Autodesk Inventor part; units mm, degrees
ref_plane "bnt_nut_1_XY" through (0, 0, 0) normal (1, 0, 0) x (0, 0, -1)
ref_plane "bnt_nut_1_YZ" through (0, 0, 0) normal (0, 0, -1) x (0, 1, 0)
ref_plane "bnt_nut_1_ZX" through (0, 0, 0) normal (0, 1, 0) x (1, 0, 0)
sketch "Sketch_1" plane through (0, 0, 0) normal (1, 0, 0) x (0, 1, 0)
  line L0 (17, 24) -> (7, 24)
  line L1 (7, 24) -> (6, 23)
  line L2 (6, 23) -> (-12, 23)
  line L3 (-19, 16) -> (-19, -16)
  line L4 (-12, -23) -> (6, -23)
  line L5 (6, -23) -> (7, -24)
  line L6 (7, -24) -> (17, -24)
  line L7 (17, -24) -> (17, -11)
  line L8 (17, -11) -> (16, -10)
  line L9 (16, -10) -> (16, 10)
  line L10 (16, 10) -> (17, 11)
  line L11 (17, 11) -> (17, 24)
  circle A0 centre (0, 0) radius 10
  line L12 (16, 0) -> (0, 0) construction
  line L13 (-12, -23) -> (-19, -16)
  line L14 (-12, 23) -> (-19, 16)
  line L15 (0, 0) -> (-19, 0) construction
  line L16 (6, 23) -> (6, -23) construction
  dimension "d39" = 20
  dimension "d41" = 46
  dimension "d43" = 23
  dimension "d45" = 1
  dimension "d46" = 48
  dimension "d47" = 1
  dimension "d48" = 36
  dimension "d49" = 10
  dimension "d50" = 10
  dimension "d51" = 20
  dimension "d52" = 13
  dimension "d53" = 13
  dimension "d54" = 32
  dimension "d55" = 16
  dimension "d56" = 135
  dimension "d57" = 18
  dimension "d58" = 18
extrude "Extrusion1" add sketch "Sketch_1" along normal blind 38
sketch "Sketch_2" plane through (29, 0, 0) normal (0.682, 0, 0.7314) x (0.7314, 0, -0.682)
  line L0 (-29, -24.55) -> (-4.4539, -24.55)
  arc A0 (-4.4539, -24.55) -> (4.4539, -24.55) centre (0, -23.4) ccw
  line L1 (4.4539, -24.55) -> (29, -24.55)
  line L2 (29, -24.55) -> (29, -23.4)
  line L3 (29, -23.4) -> (-29, -23.4)
  line L4 (-29, -23.4) -> (-29, -24.55)
  dimension "d33" = 58
  dimension "d34" = 1.15
  dimension "d35" = 24.5461
  dimension "d36" = 4.6
  dimension "d37" = 24.5461
  dimension "d38" = 1.15
extrude "Extrusion2" [suppressed]
sketch "Sketch_3" plane through (0, -23.4, 0) normal (0, 1, 0) x (1, 0, 0)
  line L0 (-29, -58) -> (87, -58)
  line L1 (87, -58) -> (87, 58)
  line L2 (87, 58) -> (-29, 58)
  line L3 (-29, 58) -> (-29, -58)
  line L4 (9.6667, -9.44) -> (48.3333, -9.44)
  line L5 (48.3333, -9.44) -> (48.3333, 9.44)
  line L6 (48.3333, 9.44) -> (9.6667, 9.44)
  line L7 (9.6667, 9.44) -> (9.6667, -9.44)
extrude "Extrusion3" [suppressed]
sketch "Sketch_4" plane through (0, 0, 0) normal (0, 0, 1) x (1, 0, 0)
  line L0 (13.4367, -26.15) -> (13.4367, -24.55)
  line L1 (13.4367, -24.55) -> (15.4367, -24.55)
  line L2 (15.4367, -24.55) -> (15.4367, -25.75)
  arc A0 (15.0367, -26.15) -> (15.4367, -25.75) centre (15.0367, -25.75) ccw
  line L3 (15.0367, -26.15) -> (13.4367, -26.15)
  line L4 (13.4367, -26.15) -> (13.4367, -24.55)
revolve "Revolution1" [suppressed]
sketch "Sketch_5" plane through (0, 0, 0) normal (0, 0, 1) x (1, 0, 0)
  line L0 (44.5633, -26.15) -> (44.5633, -24.55)
  line L1 (44.5633, -24.55) -> (46.5633, -24.55)
  line L2 (46.5633, -24.55) -> (46.5633, -25.75)
  arc A0 (46.1633, -26.15) -> (46.5633, -25.75) centre (46.1633, -25.75) ccw
  line L3 (46.1633, -26.15) -> (44.5633, -26.15)
  line L4 (44.5633, -26.15) -> (44.5633, -24.55)
revolve "Revolution2" [suppressed]
sketch "Sketch_6" plane through (0, -26.15, 0) normal (0, 1, 0) x (1, 0, 0)
  line L0 (43.5633, 0.15) -> (43.5633, -0.15)
  line L1 (43.5633, -0.15) -> (44.4133, -0.15)
  line L2 (44.4133, -0.15) -> (44.4133, -1)
  line L3 (44.4133, -1) -> (44.7133, -1)
  line L4 (44.7133, -1) -> (44.7133, -0.15)
  line L5 (44.7133, -0.15) -> (45.5633, -0.15)
  line L6 (45.5633, -0.15) -> (45.5633, 0.15)
  line L7 (45.5633, 0.15) -> (44.7133, 0.15)
  line L8 (44.7133, 0.15) -> (44.7133, 1)
  line L9 (44.7133, 1) -> (44.4133, 1)
  line L10 (44.4133, 1) -> (44.4133, 0.15)
  line L11 (44.4133, 0.15) -> (43.5633, 0.15)
extrude "Extrusion4" [suppressed]
sketch "Sketch_7" plane through (0, -26.15, 0) normal (0, 1, 0) x (1, 0, 0)
  line L0 (12.4367, 0.15) -> (12.4367, -0.15)
  line L1 (12.4367, -0.15) -> (13.2867, -0.15)
  line L2 (13.2867, -0.15) -> (13.2867, -1)
  line L3 (13.2867, -1) -> (13.5867, -1)
  line L4 (13.5867, -1) -> (13.5867, -0.15)
  line L5 (13.5867, -0.15) -> (14.4367, -0.15)
  line L6 (14.4367, -0.15) -> (14.4367, 0.15)
  line L7 (14.4367, 0.15) -> (13.5867, 0.15)
  line L8 (13.5867, 0.15) -> (13.5867, 1)
  line L9 (13.5867, 1) -> (13.2867, 1)
  line L10 (13.2867, 1) -> (13.2867, 0.15)
  line L11 (13.2867, 0.15) -> (12.4367, 0.15)
extrude "Extrusion5" [suppressed]
sketch "Sketch8" plane through (0, -12, 23) normal (0, 0, 1) x (1, 0, 0)
  line L0 (0, 18) -> (0, 0)
  point P0 (7, 11.14)
  dimension "d61" = 7
hole "Hole1" at (7, -0.86, 23) direction (0, 0, -1) diameter 4.917 depth 14.1406 tip angle 120 countersink diameter 6 countersink angle 90
sketch "Sketch9" plane through (0, 17, -11) normal (0, 1, 0) x (1, 0, 0)
  line L0 (0, 13) -> (0, 0)
  line L1 (0, 13) -> (38, 13)
  point P0 (8, 7)
  dimension "d59" = 8
  dimension "d60" = 6
hole "Hole2" at (8, 17, -18) direction (0, -1, 0) diameter 4.134 depth 13 tip angle 120 countersink diameter 6 countersink angle 90
pattern_linear "Rectangular Pattern1" count 2 spacing 22 along (1, 0, 0) count 2 spacing 35 along (0, 0, 1) of "Hole2"
ref_plane "bnt_nut_1_XY" through (0, 0, 0) normal (1, 0, 0) x (0, 0, -1)
ref_plane "bnt_nut_1_YZ" through (0, 0, 0) normal (0, 0, -1) x (0, 1, 0)
ref_plane "bnt_nut_1_ZX" through (0, 0, 0) normal (0, 1, 0) x (1, 0, 0)
sketch "Sketch10" plane through (38, -23.4, -9.44) normal (0, 0, -1) x (-1, 0, 0)
  point P0 (38, 23.4)
sketch "Sketch11" plane through (38, 0, 0) normal (1, 0, 0) x (0, 0, -1)
  circle A0 centre (0, 0) radius 15.5
  dimension "d62" = 31
properties part number "BNT 2010-2.6 Nut"
CAD build for the part. Positions are in the model's coordinates, mm. A direction names the side the tool comes from. Round coordinates to 2 decimals unless told otherwise and drop trailing zeros. Write each loop counter-clockwise with the first axis right and the second up, starting at its lowest first coordinate (ties: lowest second). Pieces come first, ordered by that corner, then holes. Notation, with made-up numbers: (28.5, 65) -> (37.5, 65) arc R28 ccw to (37.5, 98) -> close; hole circle Ø5 at (5.5, 39.5). An arc over 180 degrees is marked (long way). Answer in a Markdown table with one row per item. Add a question column.
Item 1: Saw through at B-B, the plane x = 25. Write the cut outline in (y, z).
Item 2: Saw through at A-A, the plane z = 0. Write the cut outline in (x, y).
Item 3: Which spindle directions (+Z, -Z, +X, -X, +Y, -Y) get a long thin tool onto all of the face, cutting with end or side? Do faces 4 (the face through (32.018, 9.949, 16.552)), 5 (the face through (9.181, -1.994, 15.855)), 6 (the face through (19, 17, 17)). Say none if no direction does.
Item 4: Drill centre lines: line 1 (X direction, y = 13.5, z = 17); line 2 (Z direction, x = 17.5, y = -0.5); line 3 (Z direction, x = 30, y = 12). Where is each one in solid material? Low to high. Write a range as from..to.
Item 5: Saw through at C-C, the plane y = -0.86. Write the cut outline in (x, z), then the cut area to 3 significant figures.
Item 6: Drop flat-ended pins along their axis: pin 1 Ø2.5 at (x, z) = (8, -18) entering from +Y; pin 2 Ø3 at (x, z) = (13, -6.5) entering from +Y; pin 3 Ø4 at (x, y) = (7, -0.86) entering from -Z. Give the stop position or say it passes through.
Item 7: Saw through at D-D, the plane z = 6.5. Write the cut outline in (x, y).
Item 8: Mould opens along Y. For faces 1 (the face through (19, 16, 0)), 2 (the face through (31.834, 9.949, -17.046)), 3 (the face through (18.73, 5.38, -8.43)) say: pulls with the +Y half, pulls with the -Y half, needs draft (parallel to the pull), parting line crosses it, or undercut.
Findings below:
| question | item | result |
|---|---|---|
| 1 | outline | (-19, -16) -> (-12, -23) -> (6, -23) -> (7, -24) -> (17, -24) -> (17, -11) -> (16, -10) -> (16, 10) -> (17, 11) -> (17, 24) -> (7, 24) -> (6, 23) -> (-12, 23) -> (-19, 16) -> close; hole circle Ø20 at (0, 0) |
| 2 | outline | (0, -19) -> (38, -19) -> (38, -10) -> (0, -10) -> close; (0, 10) -> (38, 10) -> (38, 16) -> (0, 16) -> close |
| 3 | face 4 | +Y |
| 3 | face 5 | +Z |
| 3 | face 6 | +Z, -Z, +X, -X, +Y |
| 4 | line 1 | x = 0..5.93, 10.07..27.93, 32.07..38 |
| 4 | line 2 | z = -23..-9.99, 9.99..23 |
| 4 | line 3 | z = -24..-20.07, -15.93..14.93, 19.07..24 |
| 5 | outline | (0, -23) -> (38, -23) -> (38, -9.96) -> (0, -9.96) -> close; (0, 9.96) -> (4.54, 9.96) -> (4.54, 22.46) -> (4, 23) -> (0, 23) -> close; (9.46, 9.96) -> (38, 9.96) -> (38, 23) -> (10, 23) -> (9.46, 22.46) -> close |
| 5 | area | 926 mm^2 |
| 6 | pin 1 | stops at y = 3.53 |
| 6 | pin 2 | stops at y = 16 |
| 6 | pin 3 | stops at z = -23 |
| 7 | outline | (0, -19) -> (38, -19) -> (38, -7.6) -> (0, -7.6) -> close; (0, 7.6) -> (38, 7.6) -> (38, 16) -> (0, 16) -> close |
| 8 | face 1 | pulls with the +Y half |
| 8 | face 2 | needs draft |
| 8 | face 3 | undercut |
